from build123d import *

# Parameters (mm, degrees)
EXTRUDE_1_DEPTH     = 45
SKETCH_2_R          = 2.5
CUT_EXTRUDE_1_DEPTH = 79.302298817


with BuildPart() as part:
    # 草图1 → 凸台-拉伸1 (new body)
    with BuildSketch(Plane(origin=(0, 0, 0), x_dir=(0, 0, -1), z_dir=(1, 0, 0))):
        with BuildLine():
            Line((0, 0), (5, 0))
            Line((5, 0), (5, -10))
            Line((5, -10), (22.5, -10))
            Line((22.5, -10), (22.5, -60))
            Line((22.5, -60), (17.5, -60))
            Line((17.5, -60), (17.5, -50))
            Line((17.5, -50), (0, -50))
            Line((0, -50), (0, -42))
            ThreePointArc((0, -42), (12, -30), (0, -18))
            Line((0, -18), (0, 0))
        make_face()
    extrude(amount=EXTRUDE_1_DEPTH)

    # 草图2 → 切除-拉伸1 (cut, through all)
    with BuildSketch(Plane(origin=(0, 0, -22.5), x_dir=(-1, 0, 0), z_dir=(0, 0, -1))):
        with Locations(Location((-35, -55, 0), (0, 0, 90))):
            Circle(SKETCH_2_R)
        with Locations(Location((-10, -5, 0), (0, 0, 90))):
            Circle(SKETCH_2_R)
        with Locations(Location((-10, -55, 0), (0, 0, 90))):
            Circle(SKETCH_2_R)
        with Locations(Location((-35, -5, 0), (0, 0, 90))):
            Circle(SKETCH_2_R)
    extrude(amount=-CUT_EXTRUDE_1_DEPTH, mode=Mode.SUBTRACT)


solid = part.part
The model under review builds one solid part; all positions refer to its coordinate system, in mm. A direction names the side the tool comes from. Coordinates: 2 decimals unless noted, no trailing zeros. Write each loop counter-clockwise with the first axis right and the second up, starting at its lowest first coordinate (ties: lowest second). Pieces come first, ordered by that corner, then holes. Notation, with made-up numbers: (-4, 66) - (6, 66) arc R23 ccw to (6, 100) - close; hole circle Ø9 at (-25.5, 60). An arc over 180 degrees is marked (long way). Answer as CSV lines item,"result".
(1) We need section C-C (x = 34). Give the boundary of the cut face in (y, z), plus the area to 3 significant figures.
Data:
outline,"(-60, -22.5) - (-57.29, -22.5) - (-57.29, -17.5) - (-60, -17.5) - close; (-52.71, -22.5) - (-10, -22.5) - (-10, -5) - (-7.29, -5) - (-7.29, 0) - (-18, 0) arc R12 cw to (-42, 0) - (-50, 0) - (-50, -17.5) - (-52.71, -17.5) - close; (-2.71, -5) - (0, -5) - (0, 0) - (-2.71, 0) - close"
area,"728 mm2"
(2) Clearance check with flat-ended pins moving along their axes: pin 1 Ø5 at (x, y) = (23.5, -7) entering from -Z; pin 2 Ø9 at (x, z) = (15.5, -9.5) entering from -Y; pin 3 Ø5 at (x, y) = (23.5, -55.5) entering from +Z; pin 4 Ø1 at (y, z) = (-52, -8.5) entering from -X. State where each tip first meets the part, or that it passes through.
Data:
pin 1,"stops at z = -5"
pin 2,"stops at y = -50"
pin 3,"stops at z = -17.5"
pin 4,"passes through"
(3) Tool access review of faces 5 (the flat face through (22, -10, -14)), 6 (the flat face through (22, -60, -20)), 7 (the flat face through (22, -55, -17.5)): name each direction out of +Z, -Z, +X, -X, +Y, -Y from which nothing blocks a thin tool from reaching the whole face with its end or side.
Data:
face 5,"-Z, +X, -X, +Y"
face 6,"+Z, -Z, +X, -X, -Y"
face 7,"+Z, +X, -X, -Y"
(4) We need section D-D (z = -2.5). Give the boundary of the cut face in (x, y), plus the area to 3 significant figures.
Data:
outline,"(0, -50) - (45, -50) - (45, -41.74) - (0, -41.74) - close; (0, -18.26) - (45, -18.26) - (45, 0) - (0, 0) - close; hole circle Ø5 at (10, -5); hole circle Ø5 at (35, -5)"
area,"1,150 mm2"
(5) We need section B-B (y = -55). Give the boundary of the cut face in (x, z).
Data:
outline,"(0, -22.5) - (7.5, -22.5) - (7.5, -17.5) - (0, -17.5) - close; (12.5, -22.5) - (32.5, -22.5) - (32.5, -17.5) - (12.5, -17.5) - close; (37.5, -22.5) - (45, -22.5) - (45, -17.5) - (37.5, -17.5) - close"
(6) We need section A-A (z = -10.25). Give the boundary of the cut face in (x, y), plus the area to 3 significant figures.
Data:
outline,"(0, -50) - (45, -50) - (45, -36.24) - (0, -36.24) - close; (0, -23.76) - (45, -23.76) - (45, -10) - (0, -10) - close"
area,"1,240 mm2"
(7) Mouldability with a two-part tool opening along X and no side actions: class faces 1 (the flat face through (22, -5, -5)), 2 (the flat face through (45, -30, -14)), 3 (the cylindrical face through (34.04, -52.69, -20.04)), 4 (the cylindrical face through (7.78, -3.85, -2.54)) as pulls with the +X half, pulls with the -X half, needs draft (parallel to the pull), parting line crosses it, or undercut.
Data:
face 1,"needs draft"
face 2,"pulls with the +X half"
face 3,"undercut"
face 4,"undercut"
(8) For line 1 along X through (y, z) = (-5, -1.7); line 2 along Y through (x, z) = (41, -20.75); line 3 along Y through (x, z) = (24.5, -7.25), list the stretches that pass through material, from the lowest coordinate up. Write a range as [from, to].
Data:
line 1,"x = [0, 7.5], [12.5, 32.5], [37.5, 45]"
line 2,"y = [-60, -10]"
line 3,"y = [-50, -39.56], [-20.44, -10]"
